The model under review builds one solid part; all positions refer to its coordinate system, in mm. A direction names the side the tool comes from. Round coordinates to 2 decimals unless told otherwise and drop trailing zeros. Order: outer loops, then holes, each group sorted by start corner. A loop starts at its lowest first (then second) coordinate and runs counter-clockwise, first axis right, second up. Notation, with made-up numbers: (53, 61) -> (104, 61) arc R23 ccw to (104, 92) -> close; hole circle Ø10 at (19, 23.25). An arc over 180 degrees is marked (long way). Return JSON: item names as keys, results as strings. Group by question number.
from build123d import *

# Parameters (mm, degrees)
ODGI_CIE_BAZOWE1_DEPTH  = 3
OTW_R_POD_RUB_M41_D     = 4.5
OTW_R_POD_RUB_M41_DEPTH = 10
OTW_R_POD_RUB_M41_TIP   = 1.351936393
ZAOKR_GLENIE1_R         = 3


# Sheet-metal steps are written as plain solids
with BuildPart() as part:
    # Szkic1 → Odgięcie bazowe1 (new body)
    with BuildSketch(Plane(origin=(0, 0, 0), x_dir=(1, 0, 0), z_dir=(0, 1, 0))):
        Polygon((9.5, 15), (-9.5, 15), (-9.5, 0), (-30, 0), (-30, -13), (30, -13), (30, 0), (9.5, 0), align=None)
    extrude(amount=-ODGI_CIE_BAZOWE1_DEPTH)

    # Otwór pod śrubę M41
    with Locations(Plane(origin=(0, 0, 0), x_dir=(1, 0, 0), z_dir=(0, 1, 0))):
        with Locations((-5.25, 9), (5.25, 9), (-15, -6.5), (15, -6.5), (-24, -6.5), (24, -6.5)):
            Hole(OTW_R_POD_RUB_M41_D / 2, depth=OTW_R_POD_RUB_M41_DEPTH)
            with Locations((0, 0, -(OTW_R_POD_RUB_M41_DEPTH + OTW_R_POD_RUB_M41_TIP / 2))):  # 118° drill point
                Cone(0, OTW_R_POD_RUB_M41_D / 2, OTW_R_POD_RUB_M41_TIP, mode=Mode.SUBTRACT)

    # Zaokrąglenie1
    zaokr_glenie1_edges = [part.edges().sort_by_distance(p)[0] for p in [
        (-9.5, -1.5, -15),
        (9.5, -1.5, -15),
        (9.5, -1.5, 0),
        (30, -1.5, 0),
        (30, -1.5, 13),
        (-30, -1.5, 13),
        (-30, -1.5, 0),
        (-9.5, -1.5, 0),
    ]]
    fillet(zaokr_glenie1_edges, radius=ZAOKR_GLENIE1_R)


solid = part.part
Item 1: Consider section A-A on x = -5.25. State the section outline as (y, z) points.
Item 2: Consider section C-C on y = -1.6. State the section outline as (x, z) points, plus the area to 3 significant figures.
Item 3: Insertion check: pin 1 Ø7 at (x, z) = (15, 6.5) entering from -Y; pin 2 Ø1.5 at (y, z) = (-2.5, -6) entering from -X; pin 3 Ø1.5 at (x, y) = (-18, -1) entering from -Z. Each pin has a flat end and moves straight along its axis. Give the tip position at first contact, or say it passes through.
Item 4: Wall thickness on line 1 along Z through (x, y) = (-24, -1.5); line 2 along Z through (x, y) = (-5.25, -1.9); line 3 along X through (y, z) = (-2.7, 10.25): over which ranges is each line inside the solid? List them lowest first.
Item 5: Consider section B-B on z = -9. State the section outline as (x, y) points.
Item 6: The part is to be moulded in two halves that separate along Z. For faces 1 (the face through (12.854, -1.521, 5.824)), 2 (the face through (10.36, -1.52, -0.9)), 3 (the face through (4.04, -1.521, -10.897)), 4 (the face through (0, -1, 13)), say which applies: +Z half, -Z half, draft (parallel to the pull), parting line (faces both ways), or undercut.
Item 7: Consider section D-D on z = 5. State the section outline as (x, y) points.
Item 8: For faces 5 (the face through (9.5, -1, -7)), 6 (the face through (-20, -1, 0)), 7 (the face through (-26.146, -1.521, 5.824)), list the 3-axis set-ups (+Z, -Z, +X, -X, +Y, -Y) from which the entire face can be reached by the end or side of a thin tool; tool diameter is ignored.
Values:
{
 "1": {"outline": "(-3, -15) -> (0, -15) -> (0, -11.25) -> (-3, -11.25) -> close; (-3, -6.75) -> (0, -6.75) -> (0, 13) -> (-3, 13) -> close"},
 "2": {"outline": "(-30, 3) arc R3 ccw to (-27, 0) -> (-12.5, 0) arc R3 cw to (-9.5, -3) -> (-9.5, -12) arc R3 ccw to (-6.5, -15) -> (6.5, -15) arc R3 ccw to (9.5, -12) -> (9.5, -3) arc R3 cw to (12.5, 0) -> (27, 0) arc R3 ccw to (30, 3) -> (30, 10) arc R3 ccw to (27, 13) -> (-27, 13) arc R3 ccw to (-30, 10) -> close; hole circle Ø4.5 at (-24, 6.5); hole circle Ø4.5 at (-15, 6.5); hole circle Ø4.5 at (-5.25, -9); hole circle Ø4.5 at (5.25, -9); hole circle Ø4.5 at (15, 6.5); hole circle Ø4.5 at (24, 6.5)", "area": "962 mm^2"},
 "3": {"pin 1": "y = -3", "pin 2": "x = -9.5", "pin 3": "z = 0"},
 "4": {"line 1": "0 to 4.25, 8.75 to 13", "line 2": "-15 to -11.25, -6.75 to 13", "line 3": "-29.99 to 29.99"},
 "5": {"outline": "(-9.5, -3) -> (-7.5, -3) -> (-7.5, 0) -> (-9.5, 0) -> close; (-3, -3) -> (3, -3) -> (3, 0) -> (-3, 0) -> close; (7.5, -3) -> (9.5, -3) -> (9.5, 0) -> (7.5, 0) -> close"},
 "6": {"face 1": "undercut", "face 2": "-Z half", "face 3": "undercut", "face 4": "+Z half"},
 "7": {"outline": "(-30, -3) -> (-25.68, -3) -> (-25.68, 0) -> (-30, 0) -> close; (-22.32, -3) -> (-16.68, -3) -> (-16.68, 0) -> (-22.32, 0) -> close; (-13.32, -3) -> (13.32, -3) -> (13.32, 0) -> (-13.32, 0) -> close; (16.68, -3) -> (22.32, -3) -> (22.32, 0) -> (16.68, 0) -> close; (25.68, -3) -> (30, -3) -> (30, 0) -> (25.68, 0) -> close"},
 "8": {"face 5": "-Z, +X, +Y, -Y", "face 6": "-Z, -X, +Y, -Y", "face 7": "+Y, -Y"}
}
